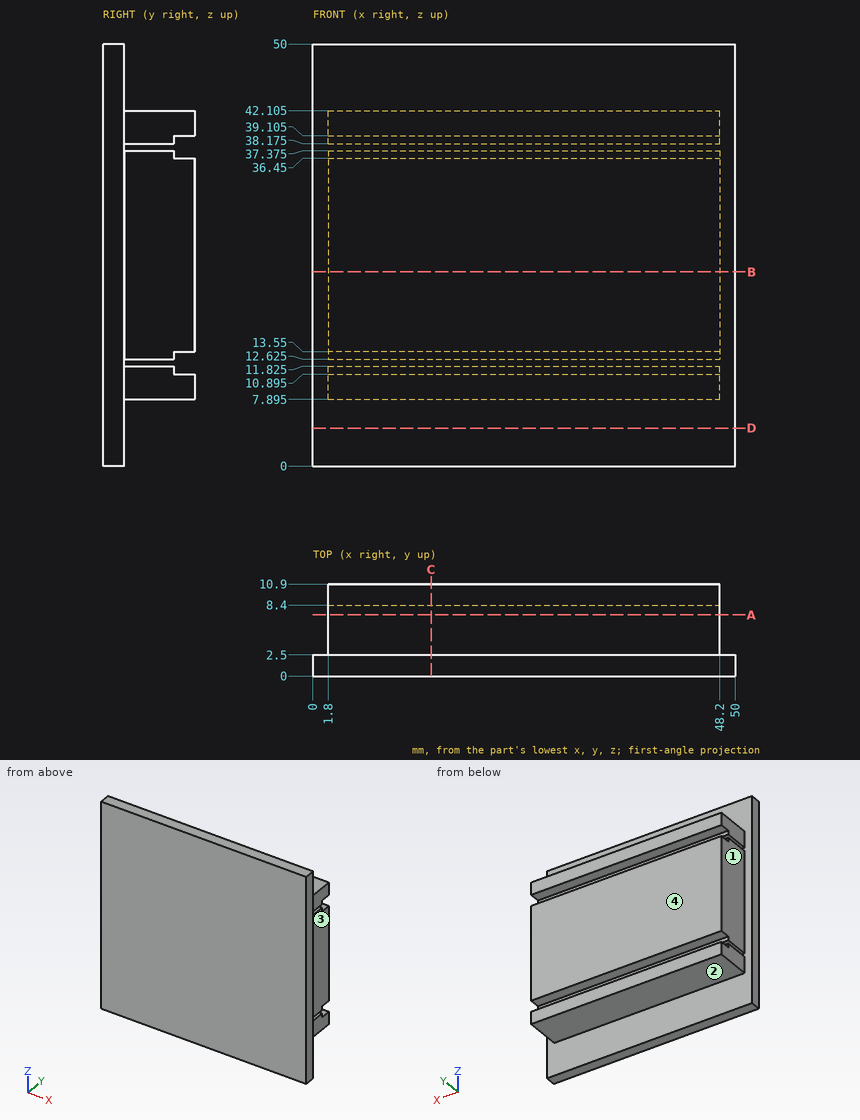
The figure shows three views and two pictorial views of one solid part (mm, origin at its lowest corner). Answer the questions. A direction names the side the tool comes from. Round coordinates to 2 decimals unless told otherwise and drop trailing zeros. Loops run counter-clockwise (first coordinate to the right, second up) from the corner with the lowest first, then second, coordinate; pieces in that order, holes last. Notation, with made-up numbers: M 68.25,-23.75 L 117.25,-23.75 A21 cw 117.25,-11.75 Z; hole C -32,-21 d7. An arc over 180 degrees is marked long. Return JSON: item names as keys, results as strings.
Q1. Find section C-C, the plane x = 14. Determine the outline of the cut face in (y, z) (3 decimals), plus the area to 3 significant figures.
Results list:
{"outline": "M 0,0 L 2.5,0 L 2.5,7.895 L 10.9,7.895 L 10.9,10.895 L 8.4,10.895 L 8.4,11.825 L 2.5,11.825 L 2.5,12.625 L 8.4,12.625 L 8.4,13.55 L 10.9,13.55 L 10.9,36.45 L 8.4,36.45 L 8.4,37.375 L 2.5,37.375 L 2.5,38.175 L 8.4,38.175 L 8.4,39.105 L 10.9,39.105 L 10.9,42.105 L 2.5,42.105 L 2.5,50 L 0,50 Z", "area": "390 mm2"}
Q2. Find section A-A, the plane y = 7.25. Determine the outline of the cut face in (x, z) (3 decimals), plus the area to 3 significant figures.
Results list:
{"outline": "M 1.8,7.895 L 48.2,7.895 L 48.2,11.825 L 1.8,11.825 Z; M 1.8,12.625 L 48.2,12.625 L 48.2,37.375 L 1.8,37.375 Z; M 1.8,38.175 L 48.2,38.175 L 48.2,42.105 L 1.8,42.105 Z", "area": "1,510 mm2"}
Q3. Find section D-D, the plane z = 4.5. Determine the outline of the cut face in (x, y), plus the area to 3 significant figures.
Results list:
{"outline": "M 0,0 L 50,0 L 50,2.5 L 0,2.5 Z", "area": "125 mm2"}
Q4. Find section B-B, the plane z = 23. Determine the outline of the cut face in (x, y), plus the area to 3 significant figures.
Results list:
{"outline": "M 0,0 L 50,0 L 50,2.5 L 48.2,2.5 L 48.2,10.9 L 1.8,10.9 L 1.8,2.5 L 0,2.5 Z", "area": "515 mm2"}
Q5. Each of these flat-tipped pins is pushed along its axis until it touches: pin 1 Ø2 at (x, y) = (30, 9) entering from -Z (3 decimals); pin 2 Ø2 at (x, y) = (17.5, 10) entering from +Z (3 decimals); pin 3 Ø3 at (y, z) = (7.5, 44) entering from -X; pin 4 Ø2 at (y, z) = (5, 9.5) entering from -X. Where does it stop, or does it pass through?
Results list:
{"pin 1": "stops at z = 7.895", "pin 2": "stops at z = 42.105", "pin 3": "passes through", "pin 4": "stops at x = 1.8"}
Q6. Which of the six approach directions +Z, -Z, +X, -X, +Y, -Y give full straight-line access (tool end or side, diameter ignored) to the marked faces 1, 2, 3 and 4?
Results list:
{"face 1": "+Z, -Z, -X, +Y", "face 2": "-Z, +X, -X, +Y", "face 3": "+Z, -Z, +X, +Y", "face 4": "+Z, -Z, +X, -X, +Y"}
Q7. Find the intervals of material crossed by line 1 along Z through (x, y) = (32, 7.25) (3 decimals); line 2 along Z through (x, y) = (15, 9.5) (3 decimals); line 3 along X through (y, z) = (9.5, 27), in increasing order. Write a range as from..to.
Results list:
{"line 1": "z = 7.895..11.825, 12.625..37.375, 38.175..42.105", "line 2": "z = 7.895..10.895, 13.55..36.45, 39.105..42.105", "line 3": "x = 1.8..48.2"}
